Autodesk Inventor part; units mm, degrees
ref_plane "Work Plane1" through (-59.5, 0, 0) normal (1, 0, 0) x (0, 0, -1)
ref_plane "YZ Plane" through (0, 0, 0) normal (1, 0, 0) x (0, 1, 0)
ref_plane "XZ Plane" through (0, 0, 0) normal (0, 1, 0) x (-1, 0, 0)
sketch "Sketch1" plane through (0, 0, 0) normal (0, 1, 0) x (-1, 0, 0)
  line L0 (0, 0) -> (119, 0)
  line L1 (119, 0) -> (119, -110.2)
  line L2 (119, -110.2) -> (0, -110.2)
  line L3 (0, -110.2) -> (0, 0)
  dimension "d0" = 119
  dimension "d1" = 110.2
extrude "Extrusion1" add sketch "Sketch1" along normal blind 2.5
sketch "Sketch2" plane through (0, 2.5, 0) normal (0, 1, 0) x (1, 0, 0)
  line L0 (-119, 0) -> (0, 0)
  line L1 (0, 0) -> (0, 110.2)
  line L2 (0, 110.2) -> (-119, 110.2)
  line L3 (-119, 110.2) -> (-119, 0)
  circle A0 centre (-114.875, 4.375) radius 1.55
  circle A1 centre (-11.5301, 10.067) radius 1.55
  circle A2 centre (-11.5301, 99.7072) radius 1.55
  circle A3 centre (-114.875, 105.95) radius 1.55
  dimension "d4" = 3.1
  dimension "d5" = 3.1
  dimension "d6" = 3.1
  dimension "d7" = 3.1
  dimension "d8" = 4.375
  dimension "d9" = 4.125
  dimension "d10" = 4.25
  dimension "d11" = 4.125
extrude "Extrusion2" cut sketch "Sketch2" against normal through all contours A0 | A3
ref_plane "Work Plane1" through (-59.5, 0, 0) normal (1, 0, 0) x (0, 0, -1)
mirror "Mirror1" about plane through (-59.5, 0, 0) normal (1, 0, 0) of "Extrusion2"
sketch "Sketch3" plane through (0, 2.5, 0) normal (0, 1, 0) x (1, 0, 0)
  circle A0 centre (-4.125, 4.375) radius 1.55
  circle A1 centre (-4.125, 105.95) radius 1.55
  circle A2 centre (-114.875, 4.375) radius 1.55
  circle A3 centre (-114.875, 105.95) radius 1.55
  line L0 (-119, 0) -> (0, 0)
  line L1 (0, 0) -> (0, 110.2)
  line L2 (0, 110.2) -> (-119, 110.2)
  line L3 (-119, 110.2) -> (-119, 0)
  circle A4 centre (-59.5, 55.1) radius 30
  circle A5 centre (-34.5, 80.1) radius 1.35
  circle A6 centre (-34.5, 30.1) radius 1.35
  circle A7 centre (-84.5, 30.1) radius 1.35
  circle A8 centre (-84.5, 80.1) radius 1.35
  dimension "d26" = 2.7
  dimension "d27" = 2.7
  dimension "d30" = 50
  dimension "d31" = 50
  dimension "d32" = 50
  dimension "d33" = 25
  dimension "d34" = 25
  dimension "d35" = 25
  dimension "d36" = 60
extrude "Extrusion3" cut sketch "Sketch3" against normal through all contours A4 | A5 | A6 | A7 | A8
properties part number "Base Cover Left"
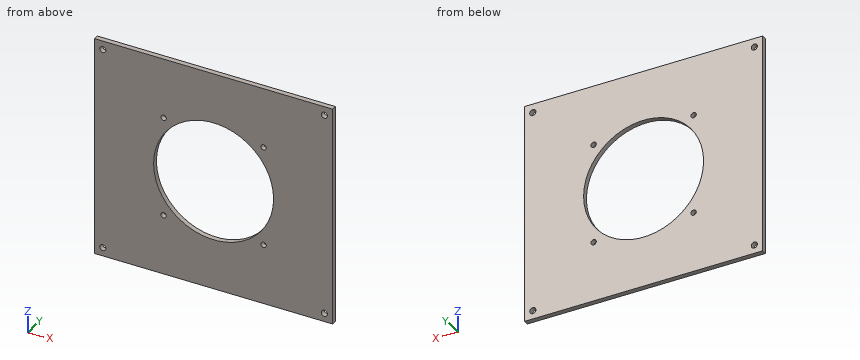
For this review, take the finished solid that the model builds, in its own axes (mm). Give positions to 0.01 mm unless a question says otherwise; leave off trailing zeros. Order: outer loops, then holes, each group sorted by start corner. A loop starts at its lowest first (then second) coordinate and runs counter-clockwise, first axis right, second up. Notation, with made-up numbers: (46.5, -2.75) - (67.5, -2.75) arc R11 cw to (67.5, 9.25) - close; hole circle Ø10 at (-25.75, 40.5). An arc over 180 degrees is marked (long way). Answer as a JSON object with one key per item and string values. Group by question number.
Item 1: Take a section at A-A on x = -59.5. Give the boundary of the cut face in (y, z), and give its area (4 significant figures).
Item 2: Wall thickness on line 1 along X through (y, z) = (0.75, -80.1); line 2 along X through (y, z) = (1.4, -106); line 3 along X through (y, z) = (0.1, -29): over which ranges is each line inside the solid? List them lowest first.
Item 3: Take a section at B-B on z = -80.1. Give the boundary of the cut face in (x, y), and give its area (3 significant figures).
Item 4: Take a section at D-D on z = -33. Give the boundary of the cut face in (x, y), and give its area (3 significant figures).
Item 5: Take a section at C-C on y = 1.1. Give the number of separate pieces and of enclosed holes in the cut face, and give its area (3 significant figures).
Reported:
{
 "1": {"outline": "(0, -110.2) - (2.5, -110.2) - (2.5, -85.1) - (0, -85.1) - close; (0, -25.1) - (2.5, -25.1) - (2.5, 0) - (0, 0) - close", "area": "125.5 mm^2"},
 "2": {"line 1": "-119 to -85.85, -83.15 to -76.08, -42.92 to -35.85, -33.15 to 0", "line 2": "-119 to -116.42, -113.33 to -5.67, -2.58 to 0", "line 3": "-119 to -85.28, -83.72 to -74.29, -44.71 to -35.28, -33.72 to 0"},
 "3": {"outline": "(-119, 0) - (-85.85, 0) - (-85.85, 2.5) - (-119, 2.5) - close; (-83.15, 0) - (-76.08, 0) - (-76.08, 2.5) - (-83.15, 2.5) - close; (-42.92, 0) - (-35.85, 0) - (-35.85, 2.5) - (-42.92, 2.5) - close; (-33.15, 0) - (0, 0) - (0, 2.5) - (-33.15, 2.5) - close", "area": "201 mm^2"},
 "4": {"outline": "(-119, 0) - (-79.79, 0) - (-79.79, 2.5) - (-119, 2.5) - close; (-39.21, 0) - (0, 0) - (0, 2.5) - (-39.21, 2.5) - close", "area": "196 mm^2"},
 "5": {"separate pieces": "1", "enclosed holes": "9", "area": "10,200 mm^2"}
}
